Source: CAD feature listing. Evaluate the final solid. Frame: model axes, mm. Face numbers are marked on the shaded views. A direction names the side the tool comes from. Round coordinates to 2 decimals unless told otherwise and drop trailing zeros. Use CSV: the item, a comma, the result in double quotes. Start each with the question number.
from build123d import *

# Parameters (mm, degrees)
SKETCH1_R           = 1.4
SKETCH1_R_2         = 4
BOSS_EXTRUDE1_DEPTH = 5
SKETCH2_R           = 0.75
CUT_EXTRUDE1_DEPTH  = 6
CUT_EXTRUDE2_START  = -4
SKETCH4_R           = 1.75
CUT_EXTRUDE2_DEPTH  = 10
CIRPATTERN1_COUNT   = 8
CUT_EXTRUDE3_DEPTH  = 2.5
FILLET1_R           = 1
CHAMFER1_SIZE       = 0.7


with BuildPart() as part:
    # Sketch1 → Boss-Extrude1 (new body, symmetric)
    with BuildSketch(Plane(origin=(0, 0, 0), x_dir=(1, 0, 0), z_dir=(0, 1, 0))):
        with BuildLine():
            Line((-9.70772888, 2.4), (-3.883091552, 25.96))
            ThreePointArc((-3.883091552, 25.96), (0, 29), (3.883091552, 25.96))
            Line((3.883091552, 25.96), (9.70772888, 2.4))
            ThreePointArc((9.70772888, 2.4), (0, -10), (-9.70772888, 2.4))
        make_face()
        with Locations((0, 25)):
            Circle(SKETCH1_R, mode=Mode.SUBTRACT)
        Circle(SKETCH1_R_2, mode=Mode.SUBTRACT)
    extrude(amount=BOSS_EXTRUDE1_DEPTH, both=True)

    # Sketch2 → Cut-Extrude1 (cut, symmetric)
    with BuildSketch(Plane(origin=(0, 0, 0), x_dir=(1, 0, 0), z_dir=(0, 1, 0))):
        with Locations((0, 7.05)):
            Circle(SKETCH2_R)
    cut_extrude1 = extrude(amount=CUT_EXTRUDE1_DEPTH, both=True, mode=Mode.SUBTRACT)

    # Sketch4 → Cut-Extrude2 (cut)
    with BuildSketch(Plane(origin=(0, 0, 0), x_dir=(1, 0, 0), z_dir=(0, 1, 0)).offset(CUT_EXTRUDE2_START)):
        with Locations((0, 7.05)):
            Circle(SKETCH4_R)
    cut_extrude2 = extrude(amount=CUT_EXTRUDE2_DEPTH, mode=Mode.SUBTRACT)

    # CirPattern1: Cut-Extrude1, Cut-Extrude2 ×8 about axis
    cirpattern1_axis = Axis((0, 0, 0), (0, 1, 0))
    for i in range(1, CIRPATTERN1_COUNT):
        add(cut_extrude1.rotate(cirpattern1_axis, i * 360 / CIRPATTERN1_COUNT), mode=Mode.SUBTRACT)
        add(cut_extrude2.rotate(cirpattern1_axis, i * 360 / CIRPATTERN1_COUNT), mode=Mode.SUBTRACT)

    # Sketch5 → Cut-Extrude3 (cut, symmetric)
    with BuildSketch(Plane(origin=(0, 0, 0), x_dir=(1, 0, 0), z_dir=(0, 1, 0))):
        with BuildLine():
            Line((-7.828813613, 10), (7.828813613, 10))
            Line((7.828813613, 10), (3.883091552, 25.96))
            ThreePointArc((3.883091552, 25.96), (0, 29), (-3.883091552, 25.96))
            Line((-3.883091552, 25.96), (-7.828813613, 10))
        make_face()
    extrude(amount=CUT_EXTRUDE3_DEPTH, both=True, mode=Mode.SUBTRACT)

    # Fillet1
    fillet1_edges = [part.edges().sort_by_distance(p)[0] for p in [
        (0, 2.5, -10),
        (5.855952582, 2.5, -17.98),
        (0, 2.5, -29),
        (6.795410216, 5, -14.18),
        (0, 5, -29),
        (-6.795410216, 5, -14.18),
        (0, 5, 10),
        (0, -5, 10),
        (-6.795410216, -5, -14.18),
        (0, -5, -29),
        (6.795410216, -5, -14.18),
        (-5.855952582, -2.5, -17.98),
        (0, -2.5, -10),
        (-7.828813613, 0, -10),
        (5.855952582, -2.5, -17.98),
        (7.828813613, 0, -10),
        (0, -2.5, -29),
        (-5.855952582, 2.5, -17.98),
    ]]
    fillet(fillet1_edges, radius=FILLET1_R)

    # Chamfer1
    chamfer1_edges = [part.edges().sort_by_distance(p)[0] for p in [
        (-1.4, -2.5, -25),
        (-1.4, 5, -25),
    ]]
    chamfer(chamfer1_edges, length=CHAMFER1_SIZE)


solid = part.part
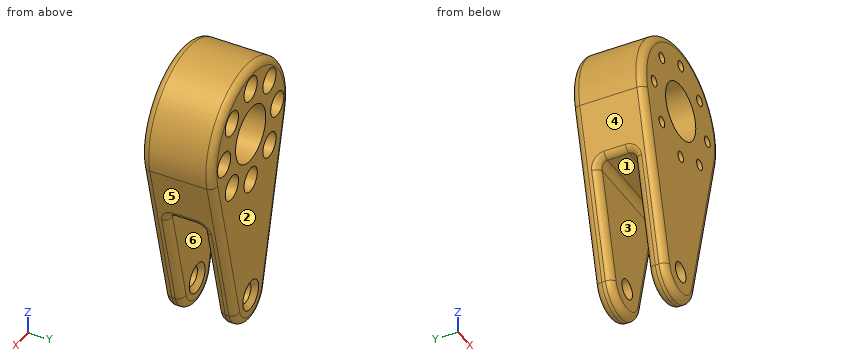
1. Reachability of the marked faces 5 and 6 from +Z, -Z, +X, -X, +Y, -Y: full face, straight path, thin tool, end or side. Return the list, or none.
2. Contact query for flat-ended pins moving along their axis: P1, Ø4, axis at x = 0, z = 8, coming from the +Y side; P2, Ø1, axis at x = -5, z = 5, coming from the +Y side; P3, Ø5, axis at y = -1.5, z = -9, coming from the -X side; P4, Ø6, axis at y = 3.5, z = 4.5, coming from the +X side. Output: stop coordinate, or through.
3. Mould query, pull axis Y, two halves, no side actions, for the marked faces 1, 2, 3 and 4. Classes: +Y half, -Y half, draft (parallel to the pull), parting line (faces both ways), or undercut.
4. Section query A-A on z = 0. Give the number of separate pieces and of enclosed holes in the cut face, and give its area (3 significant figures).
5. Line query: line 1 along X through (y, z) = (-1.5, 0); line 2 along X through (y, z) = (-4.25, -0.5); line 3 along Y through (x, z) = (0.75, -14.5). Output: solid intervals per line, ascending.
Values:
1,face 5,"-Z, +X, +Y, -Y"
1,face 6,"-Z, +X, -X"
2,P1,"stops at y = 5"
2,P2,"passes through"
2,P3,"stops at x = -8.69"
2,P4,"stops at x = 9.89"
3,face 1,"undercut"
3,face 2,"+Y half"
3,face 3,"undercut"
3,face 4,"draft"
4,separate pieces,"4"
4,enclosed holes,"0"
4,area,"53.1 mm^2"
5,line 1,"x = -10 to -8.8, -5.3 to -4, 4 to 5.3, 8.8 to 10"
5,line 2,"x = -9.96 to -7.61, -6.49 to -3.97, 3.97 to 6.49, 7.61 to 9.96"
5,line 3,"y = -5 to -2.5, 2.5 to 5"
